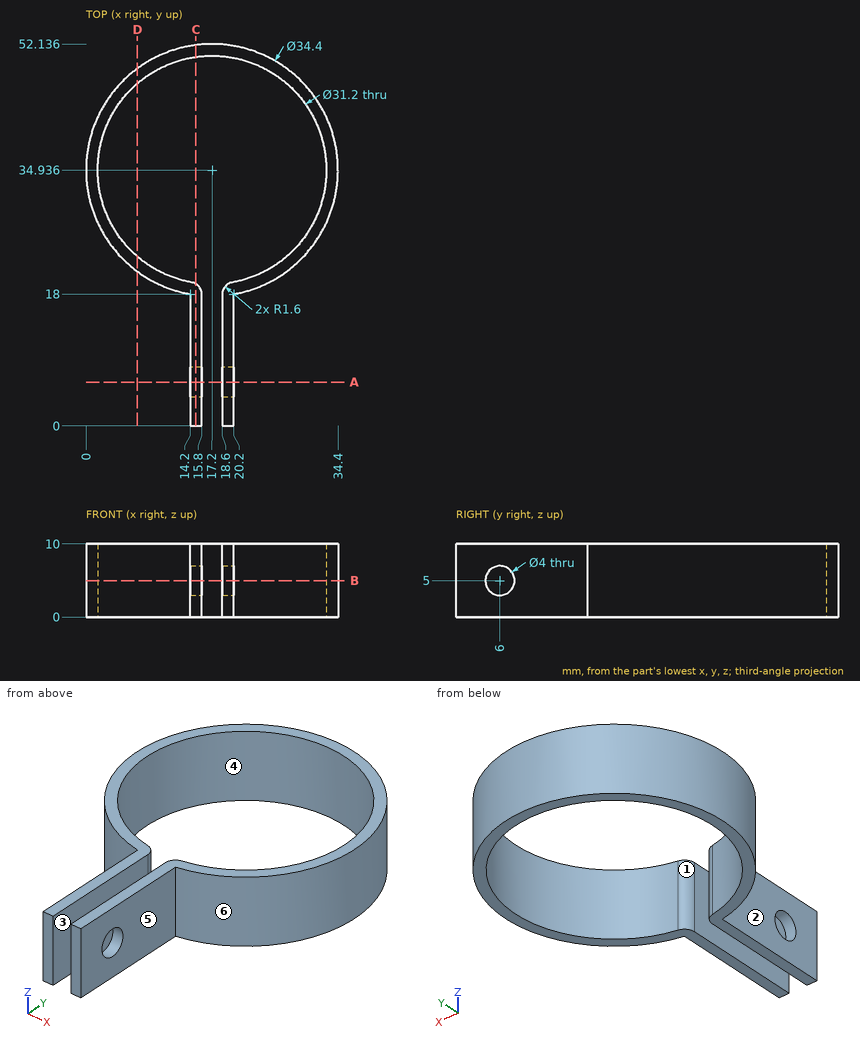
Job drawing, mm, ordinate dimensions from the low corner. One solid piece. A direction names the side the tool comes from. Give positions to 0.01 mm unless a question says otherwise; leave off trailing zeros. Write each loop counter-clockwise with the first axis right and the second up, starting at its lowest first coordinate (ties: lowest second). Pieces come first, ordered by that corner, then holes. Notation, with made-up numbers: M 76.25,-20 L 123.25,-20 A20 ccw 123.25,10 Z; hole C 34,89.25 d11. An arc over 180 degrees is marked long. Put each result on its own line as item: value. Start each with the question number.
(1) Band-saw the part on C-C, the plane x = 15. Write the cut outline in (y, z) (1 decimal).
(2) Band-saw the part on D-D, the plane x = 7. Write the cut outline in (y, z) (1 decimal).
(3) Which spindle directions (+Z, -Z, +X, -X, +Y, -Y) get a long thin tool onto all of the face, cutting with end or side? Do the marked faces 1, 2 and 3. Say none if no direction does.
(4) Probe L1, parallel to Y at x = 20, z = 4.75 (1 decimal); L2, parallel to Z at x = 19.5, y = 6; L3, parallel to X at y = 12, z = 9. List the from-to ranges inside material, lowest first.
(5) Flat gauge pins, fed straight in: pin 1 Ø5 at (x, z) = (6, 6.5) entering from +Y; pin 2 Ø5 at (y, z) = (9.5, 6) entering from +X; pin 3 Ø3 at (y, z) = (11, 7.5) entering from -X. Where does each tip first touch, or does it go through?
(6) Band-saw the part on B-B, the plane z = 5. Write the cut outline in (x, y) (1 decimal).
(7) Mould opens along Y. For the marked faces 4, 5 and 6 say: +Y half, -Y half, draft (parallel to the pull), parting line (faces both ways), or undercut.
(8) Band-saw the part on A-A, the plane y = 6. Write the cut outline in (x, z), and give its area (3 significant figures).
Response values:
1. outline: M 0,0 L 19.4,0 L 19.4,10 L 0,10 Z; M 50.4,0 L 52,0 L 52,10 L 50.4,10 Z; hole C 6,5 d4
2. outline: M 21.1,0 L 23.1,0 L 23.1,10 L 21.1,10 Z; M 46.7,0 L 48.8,0 L 48.8,10 L 46.7,10 Z
3. face 1: +Z, -Z
3. face 2: +Z, -Z, -X, -Y
3. face 3: +Z, -Z, -Y
4. L1: y = 0 to 4, 8 to 19.6, 50.3 to 51.9
4. L2: z = 0 to 3, 7 to 10
4. L3: x = 14.2 to 15.8, 18.6 to 20.2
5. pin 1: stops at y = 49.77
5. pin 2: stops at x = 20.2
5. pin 3: stops at x = 14.2
6. outline: M 14.2,0 L 15.8,0 L 15.8,4 L 14.2,4 Z; M 14.2,8 L 15.8,8 L 15.8,18 A1.6 ccw 14.5,19.6 A15.6 cw long 19.9,19.6 A1.6 ccw 18.6,18 L 18.6,8 L 20.2,8 L 20.2,18 A17.2 ccw long 14.2,18 Z; M 18.6,0 L 20.2,0 L 20.2,4 L 18.6,4 Z
7. face 4: undercut
7. face 5: draft
7. face 6: parting line
8. outline: M 14.2,0 L 15.8,0 L 15.8,3 L 14.2,3 Z; M 14.2,7 L 15.8,7 L 15.8,10 L 14.2,10 Z; M 18.6,0 L 20.2,0 L 20.2,3 L 18.6,3 Z; M 18.6,7 L 20.2,7 L 20.2,10 L 18.6,10 Z
8. area: 19.2 mm2
